Autodesk Inventor part; units mm, degrees
ref_plane "YZ Plane" through (0, 0, 0) normal (1, 0, 0) x (0, 1, 0)
ref_plane "XZ Plane" through (0, 0, 0) normal (0, 1, 0) x (-1, 0, 0)
ref_plane "XY Plane" through (0, 0, 0) normal (0, 0, 1) x (1, 0, 0)
sketch "Sketch1" plane through (0, 0, 0) normal (0, 0, 1) x (1, 0, 0)
  line L0 (-22.6695, -5.08) -> (22.6695, -5.08)
  line L1 (22.6695, -5.08) -> (22.6695, 5.08)
  line L2 (22.6695, 5.08) -> (-22.6695, 5.08)
  line L3 (-22.6695, 5.08) -> (-22.6695, -5.08)
  line L4 (-22.6695, -5.08) -> (22.6695, 5.08) construction
  line L5 (22.6695, -5.08) -> (-22.6695, 5.08) construction
  point P0 (0, 0)
  dimension "d0" = 10.16
  dimension "d1" = 45.339
extrude "Extrusion1" add sketch "Sketch1" along normal blind 5.08
sketch "Sketch2" plane through (0, 0, 0) normal (0, 0, -1) x (-1, 0, 0)
  line L0 (22.6695, 5.08) -> (22.6695, -5.08)
  line L1 (-22.6695, -5.08) -> (-22.6695, 5.08)
  line L2 (-22.6695, 5.08) -> (22.6695, 5.08)
  point P0 (0, 0)
  point P1 (18.8595, 0)
  point P2 (-18.8595, 0)
  dimension "d4" = 3.81
  dimension "d5" = 3.81
  dimension "d6" = 5.08
  dimension "d7" = 5.08
hole "Hole1" at (-18.8595, 0, 0) at (18.8595, 0, 0) direction (0, 0, 1) diameter 3.175 end through all
sketch "Sketch3" plane through (0, 0, 0) normal (0, 0, -1) x (-1, 0, 0)
  circle A0 centre (0, 0) radius 1.524
  dimension "d15" = 3.048
extrude "Extrusion2" cut sketch "Sketch3" against normal through all
sketch "Sketch4" plane through (0, 0, 5.08) normal (0, 0, 1) x (1, 0, 0)
  line L0 (22.6695, 5.08) -> (-22.6695, 5.08)
  line L1 (-22.6695, -5.08) -> (22.6695, -5.08)
  line L2 (-3.81, 5.08) -> (-8.89, 5.08)
  line L3 (-8.89, 5.08) -> (-8.89, -5.08)
  line L4 (-8.89, -5.08) -> (-3.81, -5.08)
  line L5 (-3.81, -5.08) -> (-3.81, 5.08)
  line L6 (3.81, 5.08) -> (8.89, 5.08)
  line L7 (8.89, 5.08) -> (8.89, -5.08)
  line L8 (8.89, -5.08) -> (3.81, -5.08)
  line L9 (3.81, -5.08) -> (3.81, 5.08)
  point P0 (0, 0)
  dimension "d18" = 5.08
  dimension "d19" = 3.81
  dimension "d20" = 3.81
  dimension "d21" = 5.08
extrude "Extrusion3" add sketch "Sketch4" along normal blind 12.7 contours L7 L1 L9 L0 | L5 L1 L3 L0
fillet "Fillet1" radius 3.175 2 edges at (-8.89, 0, 5.08) (8.89, 0, 5.08)
fillet "Fillet2" radius 5.08 4 edges at (6.35, -5.08, 17.78) (6.35, 5.08, 17.78) (-6.35, -5.08, 17.78) (-6.35, 5.08, 17.78)
properties part number "LowerSpringMountFrontV1nohole"
Input: part model. Units: mm. Frame: model coordinates. A direction names the side the tool comes from. Coordinates: 2 decimals unless noted, no trailing zeros. Loops run counter-clockwise (first coordinate to the right, second up) from the corner with the lowest first, then second, coordinate; pieces in that order, holes last.
Q1. Draft query along X for faces 1 (the face through (6.386, -3.553, 16.332)), 2 (the face through (8.89, 0, 13)), 3 (the face through (3.81, 0, 11)), 4 (the face through (-8.89, 0, 13)). Return one class per face: +X half, -X half, draft (parallel to the pull), parting line (faces both ways), or undercut.
Q2. Cut plane B-B (x = 0). Output: boundary loops of the cut face in (y, z), then the cut area to 3 significant figures.
Q3. Cut plane A-A (z = 12). Output: boundary loops of the cut face in (x, y).
Q4. Cut plane C-C (z = 2.25). Output: boundary loops of the cut face in (x, y) (1 decimal), then the cut area to 3 significant figures.
Q5. Set-up query: faces 5 (the face through (0, 5.08, 3)), 6 (the face through (2, 0, 5.08)), 7 (the face through (-6.314, -3.553, 16.332)), 8 (the face through (16, 0, 5.08)), 9 (the face through (-16, 0, 5.08)). Return all of +Z, -Z, +X, -X, +Y, -Y with unobstructed straight access to the full face (end or side cutting, diameter ignored); none if empty.
Q6. Material intervals for line 1 (X direction, y = 4.5, z = 10.25); line 2 (Y direction, x = 0, z = 3.7); line 3 (Z direction, x = -12, y = 3), sorted ascending.
Q7. Contact query for flat-ended pins moving along their axis: pin 1 (5 mm diameter, centred on x = -14.5, z = 5.5, fed in from -Y); pin 2 (4 mm diameter, centred on x = 18.86, y = 0, fed in from +Z); pin 3 (5 mm diameter, centred on y = 0.5, z = 14, fed in from +X); pin 4 (1.8 mm diameter, centred on x = 0, y = 0, fed in from +Z). Output: stop coordinate, or through.
Working result:
1. face 1: draft
1. face 2: +X half
1. face 3: undercut
1. face 4: -X half
2. outline: (-5.08, 0) - (-1.52, 0) - (-1.52, 5.08) - (-5.08, 5.08) - close; (1.52, 0) - (5.08, 0) - (5.08, 5.08) - (1.52, 5.08) - close
2. area: 36.1 mm2
3. outline: (-8.89, -5.08) - (-3.81, -5.08) - (-3.81, 5.08) - (-8.89, 5.08) - close; (3.81, -5.08) - (8.89, -5.08) - (8.89, 5.08) - (3.81, 5.08) - close
4. outline: (-22.7, -5.1) - (22.7, -5.1) - (22.7, 5.1) - (-22.7, 5.1) - close; hole circle Ø3.2 at (-18.9, 0); hole circle Ø3 at (0, 0); hole circle Ø3.2 at (18.9, 0)
4. area: 438 mm2
5. face 5: +Z, -Z, +X, -X, +Y
5. face 6: +Z, +Y, -Y
5. face 7: +Z, +X, -X, -Y
5. face 8: +Z, +X, +Y, -Y
5. face 9: +Z, -X, +Y, -Y
6. line 1: x = -8.89 to -3.81, 3.81 to 8.89
6. line 2: y = -5.08 to -1.52, 1.52 to 5.08
6. line 3: z = 0 to 5.08
7. pin 1: stops at y = -5.08
7. pin 2: stops at z = 5.08
7. pin 3: stops at x = 8.89
7. pin 4: passes through
